```python
from build123d import *

# Parameters (mm, degrees)
F1_DEPTH = 12.7
F0_W     = 12.7
F0_H     = 12.7
F2_DEPTH = 12.7


# Not quite as in the source:
# - ends of sketch curves that miss each other by under 0.0002 mm in the source are joined


with BuildPart() as f1:
    # F0 (on Front) → F1 (new body)
    with BuildSketch(Plane.XZ):
        Polygon((-28.6124870216, 26.0709726285), (-41.3124847398, 26.0709726285), (-41.3124847398, 13.3709726285), (-28.6124870216, 13.3709749104), align=None)
        Polygon((-41.3124847398, 38.7709726285), (-41.3124847398, 26.0709726285), (-28.6124870216, 26.0709726285), (-28.6124847398, 38.7709726285), align=None)
    extrude(amount=F1_DEPTH)

    # F0 (on Front) → F2 (join, symmetric)
    with BuildSketch(Plane.XZ):
        with Locations((-47.6624847398, 19.7209726285)):
            Rectangle(F0_W, F0_H)
        with Locations((-34.9624847398, 45.1209726285)):
            Rectangle(F0_W, F0_H)
    extrude(amount=F2_DEPTH, both=True)


solid = f1.part
```
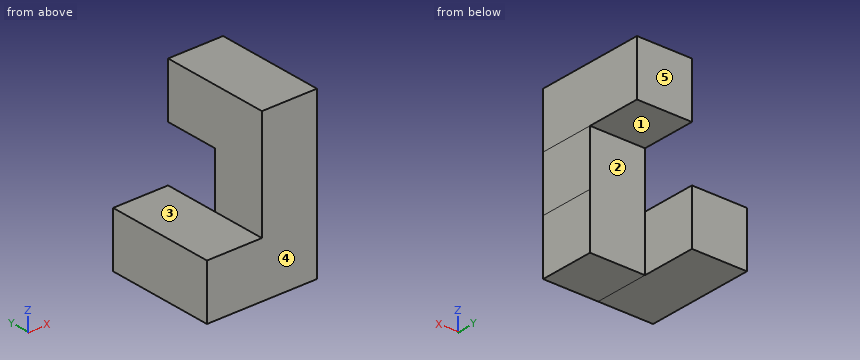
Verification items for the finished model (mm, model axes). Face numbers are marked on the shaded views. A direction names the side the tool comes from. Round coordinates to 2 decimals unless told otherwise and drop trailing zeros. Loops run counter-clockwise (first coordinate to the right, second up) from the corner with the lowest first, then second, coordinate; pieces in that order, holes last. Notation, with made-up numbers: (27.5, 34) -> (60.5, 34) arc R12 cw to (60.5, 52) -> close; hole circle Ø7 at (-8, 39.5). An arc over 180 degrees is marked (long way). Answer as a JSON object with one key per item and string values.
Q1. Section check C-C (y = -9.5). Record the boundary of the cut face in (x, z).
Data:
{"outline": "(-54.01, 13.37) -> (-41.31, 13.37) -> (-28.61, 13.37) -> (-28.61, 26.07) -> (-28.61, 38.77) -> (-28.61, 51.47) -> (-41.31, 51.47) -> (-41.31, 26.07) -> (-54.01, 26.07) -> close"}
Q2. Access from +Z, -Z, +X, -X, +Y, -Y to the whole of each face (thin tool, end or side, straight path). Record for the marked faces 1, 2, 3, 4 and 5.
Data:
{"face 1": "-Z, +X, -X, +Y", "face 2": "-Z, +X, +Y", "face 3": "+Z, -X, +Y, -Y", "face 4": "+Z, -Z, +X, -X, -Y", "face 5": "+Z, -Z, +X, -X, +Y"}
Q3. Section check B-B (x = -31.5). Record the boundary of the cut face in (y, z).
Data:
{"outline": "(-12.7, 13.37) -> (0, 13.37) -> (0, 38.77) -> (12.7, 38.77) -> (12.7, 51.47) -> (-12.7, 51.47) -> close"}
Q4. Section check A-A (y = 1.5). Record the boundary of the cut face in (x, z), then the cut area to 3 significant figures.
Data:
{"outline": "(-54.01, 13.37) -> (-41.31, 13.37) -> (-41.31, 26.07) -> (-54.01, 26.07) -> close; (-41.31, 38.77) -> (-28.61, 38.77) -> (-28.61, 51.47) -> (-41.31, 51.47) -> close", "area": "323 mm2"}
Q5. Section check D-D (z = 42). Record the boundary of the cut face in (x, y), then the cut area to 3 significant figures.
Data:
{"outline": "(-41.31, -12.7) -> (-28.61, -12.7) -> (-28.61, 12.7) -> (-41.31, 12.7) -> close", "area": "323 mm2"}
Q6. Scan lines: line 1 (X direction, y = -10, z = 49.5); line 2 (Z direction, x = -33.75, y = 10.25); line 3 (Z direction, x = -47.75, y = 6.5). Record each from-to range of solid material in increasing order. Write a range as from..to.
Data:
{"line 1": "x = -41.31..-28.61", "line 2": "z = 38.77..51.47", "line 3": "z = 13.37..26.07"}
Q7. Go/stop test with flat-tipped pins: P1, Ø5, axis at x = -46.5, y = -4.5, coming from the +Z side; P2, Ø10, axis at y = 9, z = 18, coming from the +X side; P3, Ø6.5, axis at x = -34, y = 5, coming from the -Z side; P4, Ø1.5, axis at x = -51, z = 26.5, coming from the +Y side. Record where each tip stops, or that it passes through.
Data:
{"P1": "stops at z = 26.07", "P2": "stops at x = -41.31", "P3": "stops at z = 38.77", "P4": "stops at y = 12.7"}
